from build123d import *

# Parameters (mm, degrees)
F0_W      = 30
F0_H      = 30
F1_DEPTH  = 9
F2_R      = 2.5
F3_DEPTH  = 19.6
F4_W      = 6
F4_H      = 2.5
F5_DEPTH  = 30.001
F6_R      = 1.5
F7_DEPTH  = 8
F8_R      = 1.5
F9_DEPTH  = 7.5
F11_W     = 15
F11_H     = 21.5
F12_DEPTH = 11.5


with BuildPart() as f1:
    # F0 (on Front) → F1 (new body, symmetric)
    with BuildSketch(Plane.XZ):
        Rectangle(F0_W, F0_H)
    extrude(amount=F1_DEPTH, both=True)

    # F2 (on face) → F3 (join)
    with BuildSketch(Plane(origin=(0, 0, -15), x_dir=(1, 0, 0), z_dir=(0, 0, -1))):
        with Locations((-9, 0)):
            Circle(F2_R)
        with Locations((9, 0)):
            Circle(F2_R)
    extrude(amount=F3_DEPTH)

    # F4 (on face) → F5 (cut, through all)
    with BuildSketch(Plane(origin=(-15, 0, 0), x_dir=(0, -1, 0), z_dir=(-1, 0, 0))):
        with Locations((6, 12)):
            Rectangle(F4_W, F4_H)
        with Locations((6, 8)):
            Rectangle(F4_W, F4_H)
        with Locations((6, 4)):
            Rectangle(F4_W, F4_H)
        with Locations((6, 0)):
            Rectangle(F4_W, F4_H)
        with Locations((6, -4)):
            Rectangle(F4_W, F4_H)
        with Locations((6, -8)):
            Rectangle(F4_W, F4_H)
        with Locations((6, -12)):
            Rectangle(F4_W, F4_H)
    extrude(amount=-F5_DEPTH, mode=Mode.SUBTRACT)

    # F6 (on face) → F7 (cut)
    with BuildSketch(Plane(origin=(0, 9, 0), x_dir=(-1, 0, 0), z_dir=(0, 1, 0))):
        with Locations((0, -5)):
            Circle(F6_R)
        with Locations((-4.5, 5)):
            Circle(F6_R)
        with Locations((4.5, 5)):
            Circle(F6_R)
    extrude(amount=-F7_DEPTH, mode=Mode.SUBTRACT)

    # F8 (on face) → F9 (cut)
    with BuildSketch(Plane.XY.offset(15)):
        with Locations((0, 6)):
            Circle(F8_R)
        with Locations((8.5, -6)):
            Circle(F8_R)
        with Locations((-8.5, -6)):
            Circle(F8_R)
    extrude(amount=-F9_DEPTH, mode=Mode.SUBTRACT)

    # F11 (on offset) → F12 (join)
    with BuildSketch(Plane(origin=(0, 0, -17.1), x_dir=(1, 0, 0), z_dir=(0, 0, -1))):
        with Locations((-9.5, 1.75)):
            Rectangle(F11_W, F11_H)
        with Locations((9.5, 1.75)):
            Rectangle(F11_W, F11_H)
    extrude(amount=F12_DEPTH)


solid = f1.part
Could you check a few things on this model? Use its own coordinates, in mm. A direction names the side the tool comes from. Coordinates: 2 decimals unless noted, no trailing zeros. Loops run counter-clockwise (first coordinate to the right, second up) from the corner with the lowest first, then second, coordinate; pieces in that order, holes last. Notation, with made-up numbers: (-1, 26) -> (12, 26) arc R33 ccw to (12, 58) -> close; hole circle Ø11 at (-10, 25). An arc over 180 degrees is marked (long way). Answer in a Markdown table with one row per item.
(1) Imagine slicing it at C-C (z = -7.5). List the corners of the cut face in (x, y) for me, plus the area to 3 significant figures.
Results found:
| item | result |
|---|---|
| outline | (-15, -3) -> (15, -3) -> (15, 9) -> (-15, 9) -> close |
| area | 360 mm^2 |
(2) Thinking about a two-plate mould opening in X: for faces 1 (the face through (-10, -6, 14)), 2 (the face through (-9, 0, -34.6)), which applies, released by +X, released by -X, zero draft, split by the parting line, or undercut?
Results found:
| item | result |
|---|---|
| face 1 | undercut |
| face 2 | zero draft |
(3) For faces 3 (the face through (9, -12.5, -23)), 4 (the face through (0, -6, -10.75)), 5 (the face through (0, -9, -2)), which set-ups out of +Z, -Z, +X, -X, +Y, -Y let a thin tool reach every point of the face, with its end or its side?
Results found:
| item | result |
|---|---|
| face 3 | +Z, -Z, +X, -X, -Y |
| face 4 | +X, -X, -Y |
| face 5 | +Z, +X, -X, -Y |
(4) Imagine slicing it at A-A (z = -27). List the corners of the cut face in (x, y) for me.
Results found:
| item | result |
|---|---|
| outline | (-17, -12.5) -> (-2, -12.5) -> (-2, 9) -> (-17, 9) -> close; (2, -12.5) -> (17, -12.5) -> (17, 9) -> (2, 9) -> close |
(5) Imagine slicing it at B-B (y = 0). List the corners of the cut face in (x, z) for me.
Results found:
| item | result |
|---|---|
| outline | (-17, -28.6) -> (-11.5, -28.6) -> (-11.5, -34.6) -> (-6.5, -34.6) -> (-6.5, -28.6) -> (-2, -28.6) -> (-2, -17.1) -> (-6.5, -17.1) -> (-6.5, -15) -> (6.5, -15) -> (6.5, -17.1) -> (2, -17.1) -> (2, -28.6) -> (6.5, -28.6) -> (6.5, -34.6) -> (11.5, -34.6) -> (11.5, -28.6) -> (17, -28.6) -> (17, -17.1) -> (11.5, -17.1) -> (11.5, -15) -> (15, -15) -> (15, 15) -> (-15, 15) -> (-15, -15) -> (-11.5, -15) -> (-11.5, -17.1) -> (-17, -17.1) -> close |
(6) If I drill on probe 1 along Z at (x, y) = (-4.5, 7.5); probe 2 along Z at (x, y) = (9, 7.25); probe 3 along X at (y, z) = (-4.25, -20.5), over which ranges is the centre line in solid material (lowest first)?
Results found:
| item | result |
|---|---|
| probe 1 | z = -28.6 to -17.1, -15 to 3.5, 6.5 to 15 |
| probe 2 | z = -28.6 to -17.1, -15 to 15 |
| probe 3 | x = -17 to -2, 2 to 17 |
(7) Will these pins go through, and if not, where does the flat tip stop? pin 1 Ø4 at (x, y) = (12.5, -7.5) entering from -Z; pin 2 Ø2.5 at (x, z) = (4.5, 5) entering from -Y; pin 3 Ø2.5 at (x, y) = (-8.5, -6) entering from +Z; pin 4 Ø1 at (x, z) = (13.5, -16) entering from +Y.
Results found:
| item | result |
|---|---|
| pin 1 | stops at z = -28.6 |
| pin 2 | stops at y = -9 |
| pin 3 | stops at z = 6.75 |
| pin 4 | passes through |
(8) Imagine slicing it at D-D (x = 8.5). Give the number of separate pieces and of enclosed holes in the cut face, plus the area to 3 significant figures.
Results found:
| item | result |
|---|---|
| separate pieces | 3 |
| enclosed holes | 0 |
| area | 712 mm^2 |
